The listing builds one solid part. Answer for the finished solid, in the listing's coordinates (mm). A direction names the side the tool comes from. Give positions to 0.01 mm unless a question says otherwise; leave off trailing zeros. Write each loop counter-clockwise with the first axis right and the second up, starting at its lowest first coordinate (ties: lowest second). Pieces come first, ordered by that corner, then holes. Notation, with made-up numbers: (-35, -40) - (19, -40) arc R18 cw to (19, -16) - close; hole circle Ø4 at (52.5, 63.25). An arc over 180 degrees is marked (long way). Return JSON: item names as keys, results as strings.
from build123d import *

# Parameters (mm, degrees)
F0_W      = 127
F0_H      = 127
F1_DEPTH  = 127
F2_R      = 12.7
F3_DEPTH  = 6.35
F4_R      = 12.7
F5_DEPTH  = 6.35
F6_R      = 12.7
F7_DEPTH  = 6.35
F8_R      = 12.7
F9_DEPTH  = 6.35
F11_DEPTH = 6.35
F12_R     = 12.7
F13_DEPTH = 6.35


with BuildPart() as f1:
    # F0 (on Top) → F1 (new body)
    with BuildSketch(Plane.XY):
        with Locations((63.5, 63.5)):
            Rectangle(F0_W, F0_H)
    extrude(amount=F1_DEPTH)

    # F2 (on face) → F3 (cut)
    with BuildSketch(Plane.XY.offset(127)):
        with Locations((63.000895, 61.254025)):
            Circle(F2_R)
    extrude(amount=-F3_DEPTH, mode=Mode.SUBTRACT)

    # F4 (on face) → F5 (cut)
    with BuildSketch(Plane(origin=(0, 0, 0), x_dir=(1, 0, 0), z_dir=(0, 0, -1))):
        with Locations((22.225, -22.225)):
            Circle(F4_R)
        with Locations((22.225, -63.5)):
            Circle(F4_R)
        with Locations((22.225, -104.775)):
            Circle(F4_R)
        with Locations((104.775, -63.5)):
            Circle(F4_R)
        with Locations((104.775, -22.225)):
            Circle(F4_R)
        with Locations((104.775, -104.775)):
            Circle(F4_R)
    extrude(amount=-F5_DEPTH, mode=Mode.SUBTRACT)

    # F6 (on face) → F7 (cut)
    with BuildSketch(Plane(origin=(0, 0, 0), x_dir=(0, -1, 0), z_dir=(-1, 0, 0))):
        with Locations((-22.225, 22.225)):
            Circle(F6_R)
        with Locations((-104.775, 104.775)):
            Circle(F6_R)
    extrude(amount=-F7_DEPTH, mode=Mode.SUBTRACT)

    # F8 (on face) → F9 (cut)
    with BuildSketch(Plane.YZ.offset(127)):
        with Locations((22.225, 104.775)):
            Circle(F8_R)
        with Locations((63.5, 63.5)):
            Circle(F8_R)
        with Locations((22.225, 22.225)):
            Circle(F8_R)
        with Locations((104.775, 104.775)):
            Circle(F8_R)
        with Locations((104.775, 22.225)):
            Circle(F8_R)
    extrude(amount=-F9_DEPTH, mode=Mode.SUBTRACT)

    # F10 (on face) → F11 (cut)
    with BuildSketch(Plane(origin=(0, 127, 0), x_dir=(-1, 0, 0), z_dir=(0, 1, 0))):
        with BuildLine():
            ThreePointArc((-95.794744, 31.205256), (-113.755256, 31.205256), (-113.755256, 13.244744))
            Line((-113.755256, 13.244744), (-95.794744, 31.205256))
        make_face()
        with BuildLine():
            ThreePointArc((-13.244744, 113.755256), (-31.205256, 113.755256), (-31.205256, 95.794744))
            Line((-31.205256, 95.794744), (-13.244744, 113.755256))
        make_face()
        with BuildLine():
            Line((-13.244744, 113.755256), (-31.205256, 95.794744))
            ThreePointArc((-31.205256, 95.794744), (-17.36492, 93.04173), (-9.525, 104.775))
            ThreePointArc((-9.525, 104.775), (-10.49173, 109.63508), (-13.244744, 113.755256))
        make_face()
        with BuildLine():
            ThreePointArc((-54.519744, 72.480256), (-72.480256, 72.480256), (-72.480256, 54.519744))
            Line((-72.480256, 54.519744), (-54.519744, 72.480256))
        make_face()
        with BuildLine():
            Line((-54.519744, 72.480256), (-72.480256, 54.519744))
            ThreePointArc((-72.480256, 54.519744), (-58.63992, 51.76673), (-50.8, 63.5))
            ThreePointArc((-50.8, 63.5), (-51.76673, 68.36008), (-54.519744, 72.480256))
        make_face()
        with BuildLine():
            Line((-95.794744, 31.205256), (-113.755256, 13.244744))
            ThreePointArc((-113.755256, 13.244744), (-99.91492, 10.49173), (-92.075, 22.225))
            ThreePointArc((-92.075, 22.225), (-93.04173, 27.08508), (-95.794744, 31.205256))
        make_face()
    extrude(amount=-F11_DEPTH, mode=Mode.SUBTRACT)

    # F12 (on face) → F13 (cut)
    with BuildSketch(Plane.XZ):
        with Locations((22.225, 22.225)):
            Circle(F12_R)
        with Locations((22.225, 104.775)):
            Circle(F12_R)
        with Locations((104.775, 104.775)):
            Circle(F12_R)
        with Locations((104.775, 22.225)):
            Circle(F12_R)
    extrude(amount=-F13_DEPTH, mode=Mode.SUBTRACT)


solid = f1.part
Item 1: A cutting plane is placed at C-C on x = 63.5. Determine the outline of the cut face in (y, z), then the cut area to 3 significant figures.
Answer below:
{"outline": "(0, 0) - (127, 0) - (127, 50.8) - (120.65, 50.8) - (120.65, 76.2) - (127, 76.2) - (127, 127) - (73.94, 127) - (73.94, 120.65) - (48.56, 120.65) - (48.56, 127) - (0, 127) - close", "area": "15,800 mm²"}
Item 2: A cutting plane is placed at B-B on x = 27. Determine the outline of the cut face in (y, z).
Answer below:
{"outline": "(0, 0) - (10.46, 0) - (10.46, 6.35) - (33.99, 6.35) - (33.99, 0) - (51.73, 0) - (51.73, 6.35) - (75.27, 6.35) - (75.27, 0) - (93.01, 0) - (93.01, 6.35) - (116.54, 6.35) - (116.54, 0) - (127, 0) - (127, 93.01) - (120.65, 93.01) - (120.65, 116.54) - (127, 116.54) - (127, 127) - (0, 127) - (0, 116.54) - (6.35, 116.54) - (6.35, 93.01) - (0, 93.01) - (0, 33.99) - (6.35, 33.99) - (6.35, 10.46) - (0, 10.46) - close"}
Item 3: A cutting plane is placed at A-A on y = 63.5. Determine the outline of the cut face in (x, z) (3 decimals), then the cut area to 3 significant figures.
Answer below:
{"outline": "(0, 0) - (9.525, 0) - (9.525, 6.35) - (34.925, 6.35) - (34.925, 0) - (92.075, 0) - (92.075, 6.35) - (117.475, 6.35) - (117.475, 0) - (127, 0) - (127, 50.8) - (120.65, 50.8) - (120.65, 76.2) - (127, 76.2) - (127, 127) - (75.501, 127) - (75.501, 120.65) - (50.501, 120.65) - (50.501, 127) - (0, 127) - close", "area": "15,500 mm²"}
Item 4: For faces 4 (the face through (19.472, 3.131, 9.827)), 5 (the face through (105, 120.65, 22)), 6 (the face through (22, 22, 6.35)), determine the directions among +Z, -Z, +X, -X, +Y, -Y from which every point of the face is accessible in a straight line to the end or side of a thin tool.
Answer below:
{"face 4": "-Y", "face 5": "+Y", "face 6": "-Z"}
Item 5: A cutting plane is placed at D-D on y = 15.5. Determine the outline of the cut face in (x, z), then the cut area to 3 significant figures.
Answer below:
{"outline": "(0, 0) - (11.45, 0) - (11.45, 6.35) - (33, 6.35) - (33, 0) - (94, 0) - (94, 6.35) - (115.55, 6.35) - (115.55, 0) - (127, 0) - (127, 11.45) - (120.65, 11.45) - (120.65, 33) - (127, 33) - (127, 94) - (120.65, 94) - (120.65, 115.55) - (127, 115.55) - (127, 127) - (0, 127) - (0, 33) - (6.35, 33) - (6.35, 11.45) - (0, 11.45) - close", "area": "15,400 mm²"}
Item 6: Consider L1, parallel to X at y = 63.5, z = 2.75 (3 decimals); L2, parallel to X at y = 100, z = 104; L3, parallel to Z at x = 31, y = 109.5. Determine where each line is inside the solid, lowest interval first.
Answer below:
{"L1": "x = 0 to 9.525, 34.925 to 92.075, 117.475 to 127", "L2": "x = 6.35 to 120.65", "L3": "z = 6.35 to 127"}
Item 7: The mould has two halves that part along X. Classify faces 1 (the face through (116.507, 3.131, 17.361)), 2 (the face through (6.35, 22, 22)), 3 (the face through (123.869, 20.572, 117.367)): +X half, -X half, draft (parallel to the pull), parting line (faces both ways), or undercut.
Answer below:
{"face 1": "undercut", "face 2": "-X half", "face 3": "draft"}
Item 8: Flat-ended cylindrical pins translate along their axes: P1, Ø15, axis at y = 104.775, z = 104.775, coming from the +X side; P2, Ø23, axis at y = 104.775, z = 104.775, coming from the -X side; P3, Ø12, axis at x = 81, y = 78.5, coming from the -Z side; P4, Ø12.5, axis at x = 98.5, y = 63, coming from the -Z side. Find the tip coordinate at first contact, or state that the pin passes through.
Answer below:
{"P1": "stops at x = 120.65", "P2": "stops at x = 6.35", "P3": "stops at z = 0", "P4": "stops at z = 6.35"}
